from build123d import *

# Parameters (mm, degrees)
F1_DEPTH = 7
F2_SIZE  = 2


with BuildPart() as f1:
    # F0 (on Top) → F1 (new body)
    with BuildSketch(Plane.XY):
        with BuildLine():
            Line((16.5, 0), (11, 0))
            ThreePointArc((11, 0), (0, -11), (-11, 0))
            Line((-11, 0), (-16.5, 0))
            ThreePointArc((-16.5, 0), (0, -16.5), (16.5, 0))
        make_face()
        with BuildLine():
            ThreePointArc((0, 11), (7.7781745931, 7.7781745931), (11, 0))
            Line((11, 0), (16.5, 0))
            ThreePointArc((16.5, 0), (11.6672618896, 11.6672618896), (0, 16.5))
            Line((0, 16.5), (0, 11))
        make_face()
        with BuildLine():
            ThreePointArc((-11, 0), (-7.7781745931, 7.7781745931), (0, 11))
            Line((0, 11), (0, 16.5))
            ThreePointArc((0, 16.5), (-11.6672618896, 11.6672618896), (-16.5, 0))
            Line((-16.5, 0), (-11, 0))
        make_face()
        with BuildLine():
            ThreePointArc((0, 16.5), (11.6672618896, 11.6672618896), (16.5, 0))
            Line((16.5, 0), (16.5, 36))
            ThreePointArc((16.5, 36), (11.6672618896, 24.3327381104), (0, 19.5))
            Line((0, 19.5), (0, 16.5))
        make_face()
        with BuildLine():
            ThreePointArc((-16.5, 0), (-11.6672618896, 11.6672618896), (0, 16.5))
            Line((0, 16.5), (0, 19.5))
            ThreePointArc((0, 19.5), (-11.6672618896, 24.3327381104), (-16.5, 36))
            Line((-16.5, 36), (-16.5, 0))
        make_face()
        with BuildLine():
            ThreePointArc((0, 19.5), (11.6672618896, 24.3327381104), (16.5, 36))
            ThreePointArc((16.5, 36), (0, 52.5), (-16.5, 36))
            ThreePointArc((-16.5, 36), (-11.6672618896, 24.3327381104), (0, 19.5))
        make_face()
        with BuildLine():
            ThreePointArc((11, 36), (7.7781745931, 28.2218254069), (0, 25))
            ThreePointArc((0, 25), (-7.7781745931, 43.7781745931), (11, 36))
        make_face(mode=Mode.SUBTRACT)
    extrude(amount=F1_DEPTH)

    # F2
    f2_edges = [f1.edges().sort_by_distance(p)[0] for p in [
        (16.5, 18, 0),
        (16.5, 18, 7),
    ]]
    chamfer(f2_edges, length=F2_SIZE)


solid = f1.part
Geometry: final body of the model. Coordinates: model frame, mm. Round coordinates to 2 decimals unless told otherwise and drop trailing zeros. Loops run counter-clockwise (first coordinate to the right, second up) from the corner with the lowest first, then second, coordinate; pieces in that order, holes last. Notation, with made-up numbers: (-13, -38) - (14, -38) arc R21 ccw to (14, -26) - close; hole circle Ø5 at (67, 4.25). An arc over 180 degrees is marked (long way). Write each question's results on one line, items separated by ' | '. Start each with the question number.
1) Cut plane A-A on z = 1. Return loops of the section in (x, y), then the cut area to 3 significant figures.
2) Line query: probe 1 along Y at (x, z) = (-9, 2); probe 2 along Y at (x, z) = (6.5, 4.25); probe 3 along X at (y, z) = (0.5, 2.75). Output: solid intervals per line, ascending. Write a range as [from, to].
3) Cut plane D-D on x = -7. Count the separate pieces of the cut face and the enclosed holes in it, then the cut area to 3 significant figures.
4) Cut plane C-C on y = 19.5. Return loops of the section in (x, z).
5) First-contact query: P1, Ø4, axis at x = -4, y = 9, coming from the -Z side. Flat tip, straight axial feed; report the tip coordinate or a pass-through.
6) Cut plane B-B on y = 32. Return loops of the section in (x, z).
Verdict:
1) outline: (-15.5, 0) arc R15.5 ccw to (15.5, 0) - (15.5, 36) arc R15.5 ccw to (-15.5, 36) - close; hole circle Ø22 at (0, 0); hole circle Ø22 at (0, 36) | area: 1,110 mm2
2) probe 1: y = [-13.83, -6.32], [6.32, 29.68], [42.32, 49.83] | probe 2: y = [-15.17, -8.87], [8.87, 27.13], [44.87, 51.17] | probe 3: x = [-16.5, -10.99], [10.99, 16.5]
3) separate pieces: 3 | enclosed holes: 0 | area: 215 mm2
4) outline: (-16.5, 2) - (-14.5, 0) - (14.5, 0) - (16.5, 2) - (16.5, 5) - (14.5, 7) - (-14.5, 7) - (-16.5, 5) - close
5) P1: stops at z = 0
6) outline: (-16.5, 2) - (-14.5, 0) - (-10.25, 0) - (-10.25, 7) - (-14.5, 7) - (-16.5, 5) - close; (10.25, 0) - (14.5, 0) - (16.5, 2) - (16.5, 5) - (14.5, 7) - (10.25, 7) - close
